```python
from build123d import *

# Parameters (mm, degrees)
F0_W     = 202
F0_H     = 125
F0_W_2   = 60
F0_H_2   = 60
F1_DEPTH = 1.5
F2_W     = 28
F2_H     = 10
F2_R     = 6
F2_W_2   = 19
F3_DEPTH = 1.5
F4_R     = 3
F5_DEPTH = 1.5


with BuildPart() as f1:
    # F0 (on Front) → F1 (new body)
    with BuildSketch(Plane.XZ):
        with Locations((101, 62.5)):
            Rectangle(F0_W, F0_H)
        with Locations((162, 40)):
            Rectangle(F0_W_2, F0_H_2, mode=Mode.SUBTRACT)
    extrude(amount=F1_DEPTH)

    # F2 (on face) → F3 (cut, through all)
    with BuildSketch(Plane.XZ.offset(1.5)):
        with Locations((39, 20)):
            Rectangle(F2_W, F2_H)
        with Locations((39, 40)):
            Rectangle(F2_W, F2_H)
        with Locations((20, 110)):
            Circle(F2_R)
        with Locations((54.5, 110)):
            Rectangle(F2_W_2, F2_H)
    extrude(amount=-F3_DEPTH, mode=Mode.SUBTRACT)

    # F4 (on face) → F5 (cut, through all)
    with BuildSketch(Plane(origin=(0, 0, 0), x_dir=(-1, 0, 0), z_dir=(0, 1, 0))):
        with Locations((-20, 93)):
            Circle(F4_R)
        with Locations((-115, 53)):
            Circle(F4_R)
        with Locations((-20, 53)):
            Circle(F4_R)
        with Locations((-115, 93)):
            Circle(F4_R)
    extrude(amount=-F5_DEPTH, mode=Mode.SUBTRACT)


solid = f1.part
```
Build history of the part. All positions in model axes, mm. Give positions to 0.01 mm unless a question says otherwise; leave off trailing zeros. Loops run counter-clockwise (first coordinate to the right, second up) from the corner with the lowest first, then second, coordinate; pieces in that order, holes last. Notation, with made-up numbers: (89.5, 83.25) -> (143.5, 83.25) arc R11 ccw to (143.5, 96.25) -> close; hole circle Ø5 at (26, 42). An arc over 180 degrees is marked (long way). One line per question, with ' | ' between items. Start each with the question number.
1) Cut at A-A (z = 93). Give the cut face in (x, y).
2) Two-plate mould, pull along X, no slides. Class faces 1 (the flat face through (100, 0, 63)), 2 (the cylindrical face through (20.65, -0.74, 90.07)), 3 (the cylindrical face through (113.616, -0.74, 90.338)): released by +X, released by -X, zero draft, split by the parting line, or undercut.
3) Probe L1, parallel to Z at x = 20, y = -0.3; L2, parallel to X at y = -1.4, z = 20; L3, parallel to Z at x = 115, y = -0.35. List the from-to ranges inside material, lowest first.
4) Cut at B-B (x = 43). Give the cut face in (y, z).
5) Cut at C-C (z = 53). Give the cut face in (x, y), plus the area to 3 significant figures.
6) Cut at D-D (x = 173). Give the cut face in (y, z), plus the area to 3 significant figures.
Return value:
1) outline: (0, -1.5) -> (17, -1.5) -> (17, 0) -> (0, 0) -> close; (23, -1.5) -> (112, -1.5) -> (112, 0) -> (23, 0) -> close; (118, -1.5) -> (202, -1.5) -> (202, 0) -> (118, 0) -> close
2) face 1: zero draft | face 2: undercut | face 3: undercut
3) L1: 0 to 50, 56 to 90, 96 to 104, 116 to 125 | L2: 0 to 25, 53 to 132, 192 to 202 | L3: 0 to 50, 56 to 90, 96 to 125
4) outline: (-1.5, 0) -> (0, 0) -> (0, 15) -> (-1.5, 15) -> close; (-1.5, 25) -> (0, 25) -> (0, 35) -> (-1.5, 35) -> close; (-1.5, 45) -> (0, 45) -> (0, 125) -> (-1.5, 125) -> close
5) outline: (0, -1.5) -> (17, -1.5) -> (17, 0) -> (0, 0) -> close; (23, -1.5) -> (112, -1.5) -> (112, 0) -> (23, 0) -> close; (118, -1.5) -> (132, -1.5) -> (132, 0) -> (118, 0) -> close; (192, -1.5) -> (202, -1.5) -> (202, 0) -> (192, 0) -> close | area: 195 mm^2
6) outline: (-1.5, 0) -> (0, 0) -> (0, 10) -> (-1.5, 10) -> close; (-1.5, 70) -> (0, 70) -> (0, 125) -> (-1.5, 125) -> close | area: 97.5 mm^2
